The model under review builds one solid part; all positions refer to its coordinate system, in mm. Face numbers are marked on the shaded views. A direction names the side the tool comes from. Round coordinates to 2 decimals unless told otherwise and drop trailing zeros. Order: outer loops, then holes, each group sorted by start corner. A loop starts at its lowest first (then second) coordinate and runs counter-clockwise, first axis right, second up. Notation, with made-up numbers: (39.5, 47.5) -> (58.5, 47.5) arc R11 ccw to (58.5, 52.5) -> close; hole circle Ø5 at (43.25, 42.25). An arc over 180 degrees is marked (long way). Return JSON: item names as keys, results as strings. Group by question number.
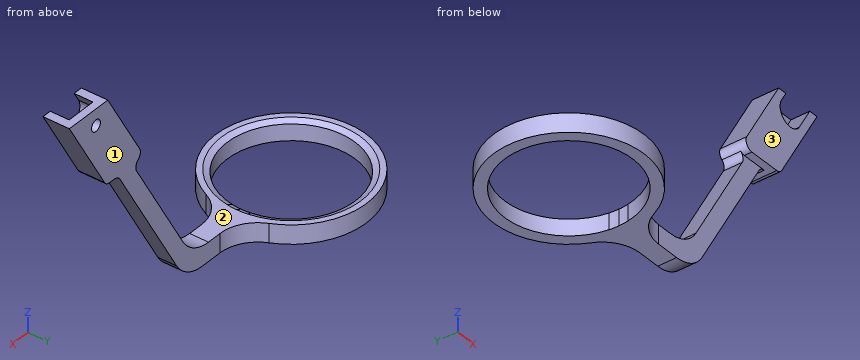
from build123d import *

# Parameters (mm, degrees)
BOSS_EXTRUDE1_DEPTH = 5
CHAMFER2_SIZE       = 1.5
CHAMFER2_SIZE2      = 0.699461487
FILLET1_R           = 10
BOSS_EXTRUDE2_DEPTH = 5
BOSS_EXTRUDE3_DEPTH = 7
CUT_EXTRUDE1_DEPTH  = 5
CUT_EXTRUDE2_DEPTH  = 1.5
SKETCH11_R          = 1.5
CUT_EXTRUDE3_DEPTH  = 102.79927269
FILLET2_R           = 10
FILLET3_R           = 2
FILLET4_R           = 2


with BuildPart() as part:
    # Sketch1 → Boss-Extrude1 (new body)
    with BuildSketch(Plane.XY):
        with BuildLine():
            ThreePointArc((16.815171721, -2.5), (-17, 0), (16.815171721, 2.5))
            Line((16.815171721, 2.5), (19.843134833, 2.5))
            ThreePointArc((19.843134833, 2.5), (-20, 0), (19.843134833, -2.5))
            Line((19.843134833, -2.5), (16.815171721, -2.5))
        make_face()
        with BuildLine():
            Line((19.843134833, 2.5), (16.815171721, 2.5))
            ThreePointArc((16.815171721, 2.5), (16.953729962, 1.253411494), (17, 0))
            ThreePointArc((17, 0), (16.953729962, -1.253411494), (16.815171721, -2.5))
            Line((16.815171721, -2.5), (19.843134833, -2.5))
            ThreePointArc((19.843134833, -2.5), (19.960745185, -1.252458251), (20, 0))
            ThreePointArc((20, 0), (19.960745185, 1.252458251), (19.843134833, 2.5))
        make_face()
        with BuildLine():
            Line((37, 2.5), (19.843134833, 2.5))
            ThreePointArc((19.843134833, 2.5), (19.960745185, 1.252458251), (20, 0))
            ThreePointArc((20, 0), (19.960745185, -1.252458251), (19.843134833, -2.5))
            Line((19.843134833, -2.5), (37, -2.5))
            Line((37, -2.5), (37, 2.5))
        make_face()
    extrude(amount=BOSS_EXTRUDE1_DEPTH)

    # Chamfer2
    chamfer2_edges = [part.edges().sort_by_distance(p)[0] for p in [
        (-16.815171721, -2.5, 5),
    ]]
    chamfer2_side = [part.faces().sort_by_distance(p)[0] for p in [
        (-17.503948469, -2.602404061, 5),
    ]]
    chamfer(chamfer2_edges, length=CHAMFER2_SIZE, length2=CHAMFER2_SIZE2, reference=chamfer2_side[0])

    # Fillet1
    fillet1_edges = [part.edges().sort_by_distance(p)[0] for p in [
        (19.843134833, 2.5, 2.5),
        (19.843134833, -2.5, 2.5),
    ]]
    fillet(fillet1_edges, radius=FILLET1_R)

    # Sketch3 → Boss-Extrude2 (add)
    with BuildSketch(Plane(origin=(0, 2.5, 0), x_dir=(1, 0, 0), z_dir=(0, 1, 0))):
        Polygon((39.113248654, 0), (74.331615075, -61), (69.331615075, -61), (37, -5), (37, 0), align=None)
    extrude(amount=-BOSS_EXTRUDE2_DEPTH)

    # Sketch5 → Boss-Extrude3 (add)
    with BuildSketch(Plane(origin=(0, 2.5, 0), x_dir=(1, 0, 0), z_dir=(0, 1, 0))):
        Polygon((65.331615075, -61), (78.331615075, -61), (65.831615075, -39.349364905), (52.831615075, -39.349364905), align=None)
    extrude(amount=-BOSS_EXTRUDE3_DEPTH)

    # Sketch9 → Cut-Extrude1 (cut)
    with BuildSketch(Plane.XZ.offset(4.5)):
        with BuildLine():
            Line((75.873066959, 61), (67.79016319, 61))
            Line((67.79016319, 61), (66.300526161, 58.419872981))
            ThreePointArc((66.300526161, 58.419872981), (67.581615075, 53.638784068), (72.362703988, 54.919872981))
            Line((72.362703988, 54.919872981), (75.873066959, 61))
        make_face()
    extrude(amount=-CUT_EXTRUDE1_DEPTH, mode=Mode.SUBTRACT)

    # Sketch10 → Cut-Extrude2 (cut)
    with BuildSketch(Plane.XZ.offset(-0.5)):
        Polygon((67.166551565, 57.919872981), (71.496678584, 55.419872981), (63.496678584, 41.563466521), (59.166551565, 44.063466521), align=None)
    extrude(amount=CUT_EXTRUDE2_DEPTH, mode=Mode.SUBTRACT)

    # Sketch11 → Cut-Extrude3 (cut, through all)
    with BuildSketch(Plane(origin=(0, 2.5, 0), x_dir=(1, 0, 0), z_dir=(0, 1, 0))):
        with Locations(Location((69.331615075, -56.669872981, 0), (0, 0, 180))):
            Circle(SKETCH11_R)
    extrude(amount=-CUT_EXTRUDE3_DEPTH, mode=Mode.SUBTRACT)

    # Fillet2
    fillet2_edges = [part.edges().sort_by_distance(p)[0] for p in [
        (37, 0, 5),
        (39.113248654, 0, 0),
    ]]
    fillet(fillet2_edges, radius=FILLET2_R)

    # Fillet3
    fillet3_edges = [part.edges().sort_by_distance(p)[0] for p in [
        (52.831615075, -1, 39.349364905),
        (65.831615075, -1, 39.349364905),
    ]]
    fillet(fillet3_edges, radius=FILLET3_R)

    # Fillet4
    # the kernel refuses this fillet: 2 mm, written as the material it adds along each edge
    with BuildSketch(Plane(origin=(61.831615075, 2.5, 39.349364905), x_dir=(1, 0, 0), z_dir=(0, -1, 0))) as fillet4_piece_1:
        with BuildLine():
            CenterArc((FILLET4_R * 0.57735026919, -FILLET4_R), FILLET4_R, 90, 60)
            Line((-FILLET4_R * 0.288675134595, -FILLET4_R * 0.5), (0, 0))
            Line((0, 0), (FILLET4_R * 0.57735026919, 0))
        make_face()
    extrude(amount=5)
    with BuildSketch(Plane(origin=(56.831615075, -2.5, 39.349364905), x_dir=(-0.9729624343176315, 0, 0.2309634200619407), z_dir=(0, 1, 0))) as fillet4_piece_2:
        with BuildLine():
            CenterArc((2.632289796, -1.822151945), FILLET4_R, 114.345531007, 82.300670054)
            Line((0.716106006, -2.395074001), (0.524487627, -2.452366207))
            Line((0.524487627, -2.452366207), (-0.191618379, -0.057292206))
            Line((-0.191618379, -0.057292206), (0.046192684, 0.194592487))
            ThreePointArc((0.046192684, 0.194592487), (0.567601681, 0.070819563), (1.725365119, 0.182215194))
            Line((1.725365119, 0.182215194), (1.807812817, 0))
        make_face()
    extrude(amount=5)


solid = part.part
Item 1: Wall thickness on line 1 along Y through (x, z) = (0, 1.1); line 2 along X through (y, z) = (0, 1.5); line 3 along Z through (x, y) = (13, 14): over which ranges is each line inside the solid? List them lowest first.
Item 2: Insertion check: pin 1 Ø12 at (x, y) = (-3, -9.5) entering from +Z; pin 2 Ø3 at (x, z) = (45.5, 10) entering from +Y; pin 3 Ø13.5 at (x, z) = (64.5, 51) entering from -Y; pin 4 Ø2 at (y, z) = (-2, 15) entering from -X. Each pin has a flat end and moves straight along its axis. Give the tip position at first contact, or say it passes through.
Item 3: Consider section D-D on z = 15.5. State the section outline as (x, y) points.
Item 4: Consider section B-B on z = 47. State the section outline as (x, y) points, plus the area to 3 significant figures.
Item 5: For the marked faces 1, 2 and 3, list the 3-axis set-ups (+Z, -Z, +X, -X, +Y, -Y) from which the entire face can be reached by the end or side of a thin tool; tool diameter is ignored.
Item 6: Consider section C-C on x = 29. State the section outline as (y, z) points.
Item 7: Consider section A-A on x = 0. State the section outline as (y, z) points, plus the area to 3 significant figures.
Values:
{
 "1": {"line 1": "-20 to -17, 17 to 20", "line 2": "-20 to -17, 17 to 38.61", "line 3": "0 to 5"},
 "2": {"pin 1": "through", "pin 2": "y = 2.5", "pin 3": "y = -4.5", "pin 4": "x = 42.2"},
 "3": {"outline": "(43.06, -2.5) -> (48.06, -2.5) -> (48.06, 2.5) -> (43.06, 2.5) -> close"},
 "4": {"outline": "(57.25, -4.5) -> (70.25, -4.5) -> (70.25, 2.5) -> (57.25, 2.5) -> close; hole (60.86, -1) -> (66.64, -1) -> (66.64, 0.5) -> (60.86, 0.5) -> close", "area": "82.3 mm^2"},
 "5": {"face 1": "+Z, -Z, +X, +Y", "face 2": "+Z, -X, +Y, -Y", "face 3": "+Z, -Z, +X, -X, -Y"},
 "6": {"outline": "(-2.5, 0) -> (2.5, 0) -> (2.5, 5) -> (-2.5, 5) -> close"},
 "7": {"outline": "(-20, 0) -> (-17, 0) -> (-17, 4.3) -> (-18.5, 5) -> (-20, 5) -> close; (17, 0) -> (20, 0) -> (20, 5) -> (18.5, 5) -> (17, 4.3) -> close", "area": "29.0 mm^2"}
}
